Could you check a few things on this model? Use its own coordinates, in mm. A direction names the side the tool comes from. Round coordinates to 2 decimals unless told otherwise and drop trailing zeros. Loops run counter-clockwise (first coordinate to the right, second up) from the corner with the lowest first, then second, coordinate; pieces in that order, holes last. Notation, with made-up numbers: (-19, 49.25) - (-8, 49.25) arc R27 cw to (-8, 78.25) - close; hole circle Ø5 at (49, 78.5). An arc over 180 degrees is marked (long way). Answer as CSV lines item,"result". Start each with the question number.
1) We'd pull the mould along X, two halves only. Please class faces 3 (the face through (595.036, -1.54, 5.742)), 4 (the face through (187.844, -1.54, -2.361)), 5 (the face through (-11, -3.038, -13)): pulls with the +X half, pulls with the -X half, needs draft (parallel to the pull), parting line crosses it, or undercut.
2) I'm going to push flat-ended pins straight in: pin 1 Ø9 at (x, z) = (-740, 775) entering from +Y; pin 2 Ø16 at (x, z) = (437.5, 200) entering from +Y; pin 3 Ø1.5 at (x, y) = (696.5, -1.5) entering from +Z; pin 4 Ø0.9 at (x, y) = (-716.5, -1.5) entering from -Z. Where does each tip first touch, or does it pass through?
3) Suppose I cut it at A-A, the plane z = -119. Write out the boundary of the cut face in (x, y), then the cut area to 3 significant figures.
4) Which directions (+Z, -Z, +X, -X, +Y, -Y) give clear straight access to the entire face, cutting with the end or side of a thin tool? Please do faces 1 (the face through (-405.88, -1.54, -50.16)), 2 (the face through (594.258, -1.54, -214.964)).
5) Please list where these lines run through material, in increasing order: line 1 along X through (y, z) = (-2.4, 890); line 2 along Z through (x, y) = (-625, -1.25); line 3 along X through (y, z) = (-1.95, -30).
6) Suppose I cut it at B-B, the plane y = -2. Count the separate pieces of the cut face and the enclosed holes in it, then the cut area to 3 significant figures.
```python
from build123d import *

# Parameters (mm, degrees)
SKETCH1_W            = 1510
SKETCH1_H            = 1810
BASE_FLANGE1_DEPTH   = 3.03784
CUT_EXTRUDE1_REACH   = 1180.584
SKETCH6_W            = 80
SKETCH6_H            = 80
M8_CLEARANCE_HOLE1_D = 10
FILLET1_R            = 10
FILLET1_OF_MIRROR1_R = 10
MIRROR2_START        = -3.03784
MIRROR2_OUTLINE_R    = 5
MIRROR2_DEPTH        = 3.03784
CUT_EXTRUDE2_REACH   = 1180.584
SKETCH12_R           = 37.5
M8_CLEARANCE_HOLE2_D = 9
FILLET2_R            = 10


# Read off the part's stored shape, not the designer's step: Mirror2
# Sheet-metal steps are written as plain solids
with BuildPart() as part:
    # Sketch1 → Base-Flange1 (new body)
    with BuildSketch(Plane(origin=(0, 0, 0), x_dir=(1, 0, 0), z_dir=(0, 1, 0))):
        Rectangle(SKETCH1_W, SKETCH1_H)
    extrude(amount=-BASE_FLANGE1_DEPTH)

    # Sketch6 → Cut-Extrude1 (cut, up to next)
    with BuildSketch(Plane(origin=(0, 0, 0), x_dir=(1, 0, 0), z_dir=(0, 1, 0)), mode=Mode.PRIVATE) as cut_extrude1_sk1:
        with Locations((-715, 865)):
            Rectangle(SKETCH6_W, SKETCH6_H)
    cut_extrude1_tool1 = extrude(cut_extrude1_sk1.sketch, amount=-CUT_EXTRUDE1_REACH, mode=Mode.PRIVATE) & part.part
    cut_extrude1 = cut_extrude1_tool1.solids().sort_by_distance((-715, 0, -865))[0]
    add(cut_extrude1, mode=Mode.SUBTRACT)

    # M8 Clearance Hole1 (through all)
    with Locations(Plane(origin=(0, -3.03784, 0), x_dir=(-1, 0, 0), z_dir=(0, -1, 0))):
        with Locations((200, 890), (200, 500), (740, 500), (740, 775), (625, 890), (437.5, 200)):
            m8_clearance_hole1 = Hole(M8_CLEARANCE_HOLE1_D / 2)

    # Fillet1
    fillet1_edges = [part.edges().sort_by_distance(p)[0] for p in [
        (-755, -1.51892, -825),
        (-675, -1.51892, -905),
        (-675, -1.51892, -825),
    ]]
    fillet(fillet1_edges, radius=FILLET1_R)

    # Mirror1: Cut-Extrude1, M8 Clearance Hole1 across plane
    add(cut_extrude1.mirror(Plane.XY), mode=Mode.SUBTRACT)
    add(m8_clearance_hole1.mirror(Plane.XY), mode=Mode.SUBTRACT)

    # Fillet1 of Mirror1
    fillet1_of_mirror1_edges = [part.edges().sort_by_distance(p)[0] for p in [
        (-755, -1.51892, 825),
        (-675, -1.51892, 905),
        (-675, -1.51892, 825),
    ]]
    fillet(fillet1_of_mirror1_edges, radius=FILLET1_OF_MIRROR1_R)

    # Mirror2 outline → Mirror2 (cut)
    with BuildSketch(Plane(origin=(0, 0, 0), x_dir=(1, 0, 0), z_dir=(0, 1, 0)).offset(MIRROR2_START)):
        with BuildLine():
            ThreePointArc((675, 835), (677.928932188, 827.928932188), (685, 825))
            Line((685, 825), (745, 825))
            ThreePointArc((745, 825), (752.071067812, 822.071067812), (755, 815))
            Line((755, 815), (755, 905))
            Line((755, 905), (665, 905))
            ThreePointArc((665, 905), (672.071067812, 902.071067812), (675, 895))
            Line((675, 895), (675, 835))
        make_face()
        with BuildLine():
            Line((755, -905), (755, -815))
            ThreePointArc((755, -815), (752.071067812, -822.071067812), (745, -825))
            Line((745, -825), (685, -825))
            ThreePointArc((685, -825), (677.928932188, -827.928932188), (675, -835))
            Line((675, -835), (675, -895))
            ThreePointArc((675, -895), (672.071067812, -902.071067812), (665, -905))
            Line((665, -905), (755, -905))
        make_face()
        with Locations((200, -890)):
            Circle(MIRROR2_OUTLINE_R)
        with Locations((200, 890)):
            Circle(MIRROR2_OUTLINE_R)
        with Locations((437.5, -200)):
            Circle(MIRROR2_OUTLINE_R)
        with Locations((437.5, 200)):
            Circle(MIRROR2_OUTLINE_R)
        with Locations((625, -890)):
            Circle(MIRROR2_OUTLINE_R)
        with Locations((625, 890)):
            Circle(MIRROR2_OUTLINE_R)
        with Locations((740, -775)):
            Circle(MIRROR2_OUTLINE_R)
        with Locations((740, 775)):
            Circle(MIRROR2_OUTLINE_R)
        with Locations((740, -500)):
            Circle(MIRROR2_OUTLINE_R)
        with Locations((740, 500)):
            Circle(MIRROR2_OUTLINE_R)
        with Locations((200, -500)):
            Circle(MIRROR2_OUTLINE_R)
        with Locations((200, 500)):
            Circle(MIRROR2_OUTLINE_R)
    extrude(amount=MIRROR2_DEPTH, mode=Mode.SUBTRACT)

    # Sketch12 → Cut-Extrude2 (cut, up to next)
    with BuildSketch(Plane.XZ.offset(3.03784), mode=Mode.PRIVATE) as cut_extrude2_sk1:
        with Locations(Location((-437.5, -30, 0), (0, 0, 270))):
            Circle(SKETCH12_R)
    cut_extrude2_tool1 = extrude(cut_extrude2_sk1.sketch, amount=-CUT_EXTRUDE2_REACH, mode=Mode.PRIVATE) & part.part
    # Sketch12 → Cut-Extrude2 (cut, up to next)
    with BuildSketch(Plane.XZ.offset(3.03784), mode=Mode.PRIVATE) as cut_extrude2_sk2:
        with Locations(Location((-162.5, -30, 0), (0, 0, 270))):
            Circle(SKETCH12_R)
    cut_extrude2_tool2 = extrude(cut_extrude2_sk2.sketch, amount=-CUT_EXTRUDE2_REACH, mode=Mode.PRIVATE) & part.part
    # Sketch12 → Cut-Extrude2 (cut, up to next)
    with BuildSketch(Plane.XZ.offset(3.03784), mode=Mode.PRIVATE) as cut_extrude2_sk3:
        with Locations(Location((162.5, -30, 0), (0, 0, 270))):
            Circle(SKETCH12_R)
    cut_extrude2_tool3 = extrude(cut_extrude2_sk3.sketch, amount=-CUT_EXTRUDE2_REACH, mode=Mode.PRIVATE) & part.part
    # Sketch12 → Cut-Extrude2 (cut, up to next)
    with BuildSketch(Plane.XZ.offset(3.03784), mode=Mode.PRIVATE) as cut_extrude2_sk4:
        with Locations(Location((437.5, -30, 0), (0, 0, 270))):
            Circle(SKETCH12_R)
    cut_extrude2_tool4 = extrude(cut_extrude2_sk4.sketch, amount=-CUT_EXTRUDE2_REACH, mode=Mode.PRIVATE) & part.part
    # Sketch12 → Cut-Extrude2 (cut, up to next)
    with BuildSketch(Plane.XZ.offset(3.03784), mode=Mode.PRIVATE) as cut_extrude2_sk5:
        with BuildLine():
            Line((755, 20), (630, 20))
            ThreePointArc((630, 20), (594.644660941, 5.355339059), (580, -30))
            Line((580, -30), (580, -180))
            ThreePointArc((580, -180), (594.644660941, -215.355339059), (630, -230))
            Line((630, -230), (755, -230))
            Line((755, -230), (755, 20))
        make_face()
    cut_extrude2_tool5 = extrude(cut_extrude2_sk5.sketch, amount=-CUT_EXTRUDE2_REACH, mode=Mode.PRIVATE) & part.part
    add(cut_extrude2_tool1.solids().sort_by_distance((-437.5, -3.03784, -30))[0], mode=Mode.SUBTRACT)
    add(cut_extrude2_tool2.solids().sort_by_distance((-162.5, -3.03784, -30))[0], mode=Mode.SUBTRACT)
    add(cut_extrude2_tool3.solids().sort_by_distance((162.5, -3.03784, -30))[0], mode=Mode.SUBTRACT)
    add(cut_extrude2_tool4.solids().sort_by_distance((437.5, -3.03784, -30))[0], mode=Mode.SUBTRACT)
    add(cut_extrude2_tool5.solids().sort_by_distance((669.419173, -3.03784, -105))[0], mode=Mode.SUBTRACT)

    # M8 Clearance Hole2 (through all)
    with Locations(Plane(origin=(0, -3.03784, 0), x_dir=(-1, 0, 0), z_dir=(0, -1, 0))):
        with Locations((-740, -37.5), (-740, 247.5), (740, 200), (740, -200), (0, 200), (0, -200)):
            Hole(M8_CLEARANCE_HOLE2_D / 2)

    # Fillet2
    fillet2_edges = [part.edges().sort_by_distance(p)[0] for p in [
        (755, -1.51892, 20),
        (755, -1.51892, -230),
    ]]
    fillet(fillet2_edges, radius=FILLET2_R)


solid = part.part
```
Filled sheet:
1,face 3,"pulls with the +X half"
1,face 4,"undercut"
1,face 5,"needs draft"
2,pin 1,"through"
2,pin 2,"y = 0"
2,pin 3,"z = 825"
2,pin 4,"z = -825"
3,outline,"(-755, -3.04) - (580, -3.04) - (580, 0) - (-755, 0) - close"
3,area,"4,060 mm²"
4,face 1,"+Y, -Y"
4,face 2,"+X, +Y, -Y"
5,line 1,"-675 to -630, -620 to -205, -195 to 195, 205 to 620, 630 to 675"
5,line 2,"-905 to -895, -885 to 885, 895 to 905"
5,line 3,"-755 to -475, -400 to -200, -125 to 125, 200 to 400, 475 to 580"
6,separate pieces,"1"
6,enclosed holes,"34"
6,area,"2,640,000 mm²"
